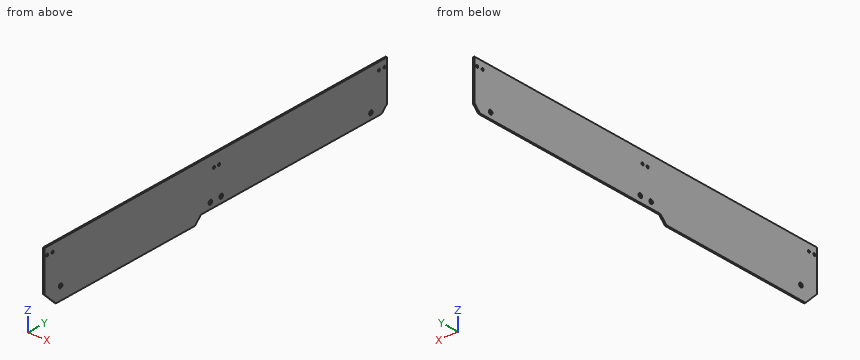
Autodesk Inventor part; units mm, degrees
ref_plane "YZ Plane" through (0, 0, 0) normal (1, 0, 0) x (0, 1, 0)
ref_plane "XZ Plane" through (0, 0, 0) normal (0, 1, 0) x (-1, 0, 0)
ref_plane "XY Plane" through (0, 0, 0) normal (0, 0, 1) x (1, 0, 0)
sketch "Sketch1" plane through (0, 0, 0) normal (1, 0, 0) x (0, 1, 0)
  line L0 (22.9119, 0) -> (-383.4881, 0)
  line L1 (-383.4881, 0) -> (-383.4881, 48.26)
  line L2 (-383.4881, 48.26) -> (22.9119, 48.26)
  line L3 (22.9119, 48.26) -> (22.9119, 0)
  line L4 (22.9119, 0) -> (22.9119, 1.6002)
  line L5 (-383.4881, 22.987) -> (-383.4881, 2.413)
  line L6 (22.2741, 48.26) -> (-5.0281, 48.26)
  circle A0 centre (3.8619, 6.35) radius 2.1463
  circle A1 centre (-364.4381, 6.35) radius 2.1463
  circle A2 centre (-173.8111, 6.35) radius 2.1463
  circle A3 centre (-186.6381, 6.35) radius 2.1463
  circle A4 centre (19.8639, 40.64) radius 1.27
  circle A5 centre (13.2599, 40.64) radius 1.27
  circle A6 centre (-176.4781, 35.8902) radius 1.27
  circle A7 centre (-182.4471, 35.8902) radius 1.27
  circle A8 centre (-380.4401, 40.64) radius 1.27
  circle A9 centre (-373.8361, 40.64) radius 1.27
  line L7 (-383.4881, 0) -> (-370.7881, 0) construction
  line L8 (22.9119, 6.35) -> (16.5619, 0)
  line L9 (-383.4881, 6.35) -> (-370.0177, -7.1204)
  line L10 (-383.4881, 6.35) -> (-364.4381, 6.35) construction
  line L11 (-370.0177, -7.1204) -> (-204.9177, -7.1204)
  line L12 (-204.9177, -7.1204) -> (-197.7973, 0)
  point P0 (0, 0)
  point P1 (-187.7276, 0)
  dimension "d0" = 4.2926
  dimension "d1" = 6.35
  dimension "d2" = 19.05
  dimension "d3" = 4.2926
  dimension "d4" = 19.05
  dimension "d5" = 6.35
  dimension "d6" = 4.2926
  dimension "d7" = 6.35
  dimension "d8" = 4.2926
  dimension "d9" = 6.35
  dimension "d10" = 196.723
  dimension "d11" = 196.85
  dimension "d12" = 2.54
  dimension "d13" = 3.048
  dimension "d14" = 7.62
  dimension "d15" = 2.54
  dimension "d16" = 7.62
  dimension "d17" = 9.652
  dimension "d18" = 2.54
  dimension "d19" = 12.3698
  dimension "d20" = 199.39
  dimension "d21" = 2.54
  dimension "d22" = 12.3698
  dimension "d23" = 5.969
  dimension "d24" = 2.54
  dimension "d25" = 7.62
  dimension "d26" = 3.048
  dimension "d27" = 2.54
  dimension "d28" = 7.62
  dimension "d29" = 9.652
  dimension "d36" = 19.05
  dimension "d37" = 45
  dimension "d38" = 165.1
  dimension "d39" = 135
  dimension "d40" = 48.26
extrude "Extrusion1" add sketch "Sketch1" along normal blind 1.5875 contours L0 L9 L1 L2 L3 L8 | L12 L11 L9 L0
properties part number "Side Guard"
Can you work these out from the model? Positions are in its coordinate system, mm. Round coordinates to 2 decimals unless told otherwise and drop trailing zeros. Loops run counter-clockwise (first coordinate to the right, second up) from the corner with the lowest first, then second, coordinate; pieces in that order, holes last. Notation, with made-up numbers: (-12, 66.25) - (43, 66.25) arc R26 cw to (43, 104.25) - close; hole circle Ø11 at (65, -33). An arc over 180 degrees is marked (long way). Answer in a Markdown table with one row per item. Add a question column.
Q1. I want a section at A-A on x = 0.4. Count the separate pieces of the cut face and the enclosed holes in it, and give its area (3 significant figures).
Q2. I need wall thicknesses on L1, parallel to Y at x = 0.25, z = 7.5; L2, parallel to Z at x = 1.25, y = -37; L3, parallel to Y at x = 1.35, z = 40. Which ranges of each line are inside material? Lowest first, please.
Q3. I want a section at B-B on y = -24. List the corners of the cut face in (x, z) for me, and give its area (3 significant figures).
A:
| question | item | result |
|---|---|---|
| 1 | separate pieces | 1 |
| 1 | enclosed holes | 10 |
| 1 | area | 20,700 mm^2 |
| 2 | L1 | -383.49 to -366.25, -362.63 to -188.45, -184.83 to -175.62, -172 to 2.05, 5.67 to 22.91 |
| 2 | L2 | 0 to 48.26 |
| 2 | L3 | -383.49 to -381.54, -379.34 to -374.93, -372.74 to 12.16, 14.36 to 18.77, 20.96 to 22.91 |
| 3 | outline | (0, 0) - (1.59, 0) - (1.59, 48.26) - (0, 48.26) - close |
| 3 | area | 76.6 mm^2 |
